For this review, use the dimensioned drawing (mm, ordinates from the lowest corner) and the shaded views. A direction names the side the tool comes from. Coordinates: 2 decimals unless noted, no trailing zeros. Loops run counter-clockwise (first coordinate to the right, second up) from the corner with the lowest first, then second, coordinate; pieces in that order, holes last. Notation, with made-up numbers: (43, -15) - (99, -15) arc R32 cw to (99, 14) - close; hole circle Ø8 at (19.25, 62). An arc over 180 degrees is marked (long way). One line per item, written item: value. Start each with the question number.
1. We need section D-D, the plane y = 46.5. Give the boundary of the cut face in (x, z).
2. We need section A-A, the plane y = 10. Count the separate pieces of the cut face and the enclosed holes in it.
3. We need section C-C, the plane z = 10.5. Give the boundary of the cut face in (x, y) (1 decimal), then the cut area to 3 significant figures.
4. Mouldability with a two-part tool opening along X and no side actions: class the marked faces 1, 2 and 3 as +X half, -X half, draft (parallel to the pull), parting line (faces both ways), or undercut.
5. Insertion check: P1, Ø3.5, axis at y = 10, z = 40, coming from the -X side; P2, Ø10, axis at x = 32.5, y = 42, coming from the -Z side; P3, Ø2, axis at x = 18.5, y = 34.5, coming from the +Z side; P4, Ø9, axis at x = 19.5, y = 24.5, coming from the +Z side. Each pin has a flat end and moves straight along its axis. Give the tip position at first contact, or say it passes through.
6. For the marked faces 4 and 5, list the 3-axis set-ups (+Z, -Z, +X, -X, +Y, -Y) from which the entire face can be reached by the end or side of a thin tool; tool diameter is ignored.
7. To check wall thickness, follow line 1 (Y direction, x = 20, z = 1.9); line 2 (Y direction, x = 2.3, z = 40); line 3 (X direction, y = 28, z = 41.5). State the ranges of each line that lie inside material, in increasing order.
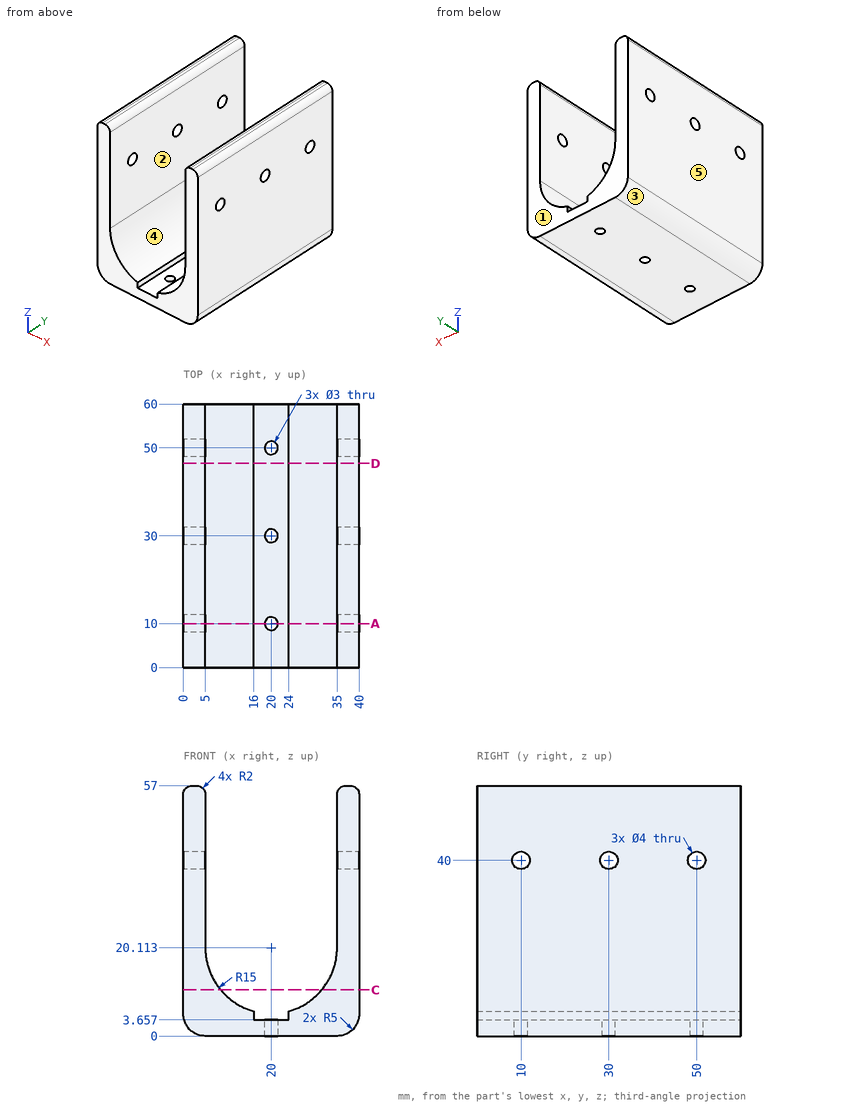
Findings below:
1. outline: (0, 5) arc R5 ccw to (5, 0) - (35, 0) arc R5 ccw to (40, 5) - (40, 55) arc R2 ccw to (38, 57) - (37, 57) arc R2 ccw to (35, 55) - (35, 20.11) arc R15 cw to (24, 5.66) - (24, 3.66) - (16, 3.66) - (16, 5.66) arc R15 cw to (5, 20.11) - (5, 55) arc R2 ccw to (3, 57) - (2, 57) arc R2 ccw to (0, 55) - close
2. separate pieces: 4
2. enclosed holes: 0
3. outline: (0, 0) - (8.5, 0) - (8.5, 60) - (0, 60) - close; (31.5, 0) - (40, 0) - (40, 60) - (31.5, 60) - close
3. area: 1,020 mm2
4. face 1: draft
4. face 2: undercut
4. face 3: -X half
5. P1: through
5. P2: z = 0
5. P3: z = 3.66
5. P4: z = 5.97
6. face 4: +Z, +Y, -Y
6. face 5: +Z, -Z, -X, +Y, -Y
7. line 1: 0 to 8.5, 11.5 to 28.5, 31.5 to 48.5, 51.5 to 60
7. line 2: 0 to 8, 12 to 28, 32 to 48, 52 to 60
7. line 3: 0 to 5, 35 to 40
